from build123d import *

# Parameters (mm, degrees)
SKETCH1_R           = 10
BOSS_EXTRUDE1_DEPTH = 50
SKETCH2_W           = 50
SKETCH2_H           = 20
CUT_EXTRUDE1_DEPTH  = 106.651549918
FILLET1_R           = 25
FILLET2_R           = 25
FILLET3_R           = 25
FILLET4_R           = 25
SKETCH3_R           = 10
CUT_EXTRUDE2_DEPTH  = 106.651549918


with BuildPart() as part:
    # Sketch1 → Boss-Extrude1 (new body)
    with BuildSketch(Plane(origin=(0, 0, 0), x_dir=(1, 0, 0), z_dir=(0, 1, 0))):
        with BuildLine():
            Line((-78.5, -15.188404139), (-78.5, -30.188404139))
            Line((-78.5, -30.188404139), (46.5, -30.188404139))
            ThreePointArc((46.5, -30.188404139), (71.5, -5.188404139), (46.5, 19.811595861))
            Line((46.5, 19.811595861), (-78.5, 19.811595861))
            Line((-78.5, 19.811595861), (-78.5, 4.811595861))
            Line((-78.5, 4.811595861), (-28.5, 4.811595861))
            Line((-28.5, 4.811595861), (-28.5, -15.188404139))
            Line((-28.5, -15.188404139), (-78.5, -15.188404139))
        make_face()
        with Locations(Location((46.5, -5.188404139, 0), (0, 0, 270))):
            Circle(SKETCH1_R, mode=Mode.SUBTRACT)
    extrude(amount=BOSS_EXTRUDE1_DEPTH)

    # Sketch2 → Cut-Extrude1 (cut, through all)
    with BuildSketch(Plane.XY.offset(30.188404139)):
        with Locations((46.5, 25)):
            Rectangle(SKETCH2_W, SKETCH2_H)
    extrude(amount=-CUT_EXTRUDE1_DEPTH, mode=Mode.SUBTRACT)

    # Fillet1
    fillet1_edges = [part.edges().sort_by_distance(p)[0] for p in [
        (-78.5, 0, -12.311595861),
    ]]
    fillet(fillet1_edges, radius=FILLET1_R)

    # Fillet2
    fillet2_edges = [part.edges().sort_by_distance(p)[0] for p in [
        (-78.5, 0, 22.688404139),
    ]]
    fillet(fillet2_edges, radius=FILLET2_R)

    # Fillet3
    fillet3_edges = [part.edges().sort_by_distance(p)[0] for p in [
        (-78.5, 50, 22.688404139),
    ]]
    fillet(fillet3_edges, radius=FILLET3_R - 0.0001)  # a hair under: the kernel refuses the full size

    # Fillet4
    fillet4_edges = [part.edges().sort_by_distance(p)[0] for p in [
        (-78.5, 50, -12.311595861),
    ]]
    fillet(fillet4_edges, radius=FILLET4_R - 0.0001)  # a hair under: the kernel refuses the full size

    # Sketch3 → Cut-Extrude2 (cut, through all)
    with BuildSketch(Plane(origin=(0, 0, -19.811595861), x_dir=(-1, 0, 0), z_dir=(0, 0, -1))):
        with Locations((53.5, 25)):
            Circle(SKETCH3_R)
    extrude(amount=-CUT_EXTRUDE2_DEPTH, mode=Mode.SUBTRACT)


solid = part.part
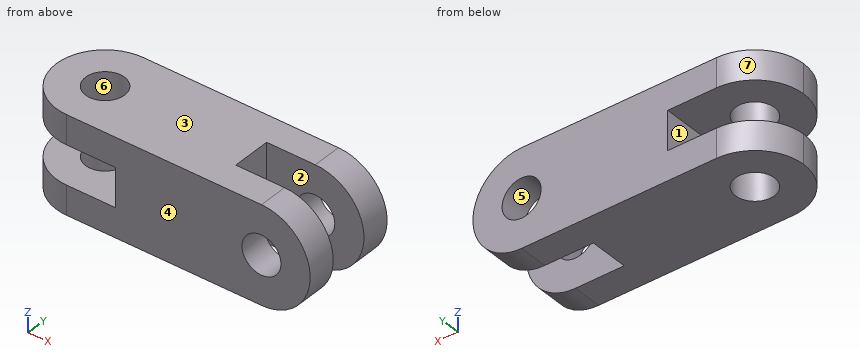
Part model, mm, in its own coordinate system. Face numbers are marked on the shaded views. A direction names the side the tool comes from. Coordinates: 2 decimals unless noted, no trailing zeros. Order: outer loops, then holes, each group sorted by start corner. A loop starts at its lowest first (then second) coordinate and runs counter-clockwise, first axis right, second up.
(1) Probe L1, parallel to Z at x = -58.5, y = 43.5; L2, parallel to Y at x = 51, z = -14; L3, parallel to X at y = 32, z = 7.5. List the from-to ranges inside material, lowest first.
Check sheet entries:
L1: z = -19.81 to -4.81, 15.19 to 30.19
L2: y = 0 to 15, 35 to 50
L3: x = -28.5 to 21.5
(2) Slice it at A-A, the plane y = 28. Write the cut outline in (x, z).
Check sheet entries:
outline: (-78.32, -19.81) - (-63.04, -19.81) - (-63.04, -4.81) - (-78.32, -4.81) - close; (-78.32, 15.19) - (-63.04, 15.19) - (-63.04, 30.19) - (-78.32, 30.19) - close; (-43.96, -19.81) - (21.5, -19.81) - (21.5, 30.19) - (-43.96, 30.19) - (-43.96, 15.19) - (-28.5, 15.19) - (-28.5, -4.81) - (-43.96, -4.81) - close
(3) Pin check, flat tips, straight feed: pin 1 Ø5 at (y, z) = (33, -8) entering from +X; pin 2 Ø25 at (x, z) = (48, 6.5) entering from +Y; pin 3 Ø16 at (y, z) = (14.5, 10) entering from -X; pin 4 Ø22 at (y, z) = (28.5, 7) entering from +X. Stop position of each tip, or through.
Check sheet entries:
pin 1: stops at x = 68.6
pin 2: stops at y = 50
pin 3: stops at x = -78.11
pin 4: stops at x = 71.5
(4) Slice it at C-C, the plane x = 49.5. Write the cut outline in (y, z).
Check sheet entries:
outline: (0, -19.63) - (15, -19.63) - (15, -4.35) - (0, -4.35) - close; (0, 14.73) - (15, 14.73) - (15, 30.01) - (0, 30.01) - close; (35, -19.63) - (50, -19.63) - (50, -4.35) - (35, -4.35) - close; (35, 14.73) - (50, 14.73) - (50, 30.01) - (35, 30.01) - close
(5) Slice it at D-D, the plane y = 38.5. Write the cut outline in (x, z), and give its area (3 significant figures).
Check sheet entries:
outline: (-74.54, -19.81) - (46.5, -19.81) arc R25 ccw to (46.5, 30.19) - (-74.54, 30.19) - (-74.54, 15.19) - (-28.5, 15.19) - (-28.5, -4.81) - (-74.54, -4.81) - close; hole circle Ø20 at (46.5, 5.19)
area: 5,800 mm2
(6) Tool access for the marked faces 1, 2 and 3: list every direction of +Z, -Z, +X, -X, +Y, -Y with a clear straight run to the whole face (end or side of a thin tool).
Check sheet entries:
face 1: -X, +Y, -Y
face 2: +Z, -Z, +X
face 3: +Z, +X, -X, +Y, -Y
(7) Pull direction X, two halves, no side cores. Call the marked faces 4, 5, 6 and 7: pulls with the +X half, pulls with the -X half, needs draft (parallel to the pull), parting line crosses it, or undercut.
Check sheet entries:
face 4: needs draft
face 5: undercut
face 6: undercut
face 7: pulls with the -X half
